The figure shows three views and two pictorial views of one solid part (mm, origin at its lowest corner). Answer the questions. A direction names the side the tool comes from. Coordinates: 2 decimals unless noted, no trailing zeros. Loops run counter-clockwise (first coordinate to the right, second up) from the corner with the lowest first, then second, coordinate; pieces in that order, holes last.
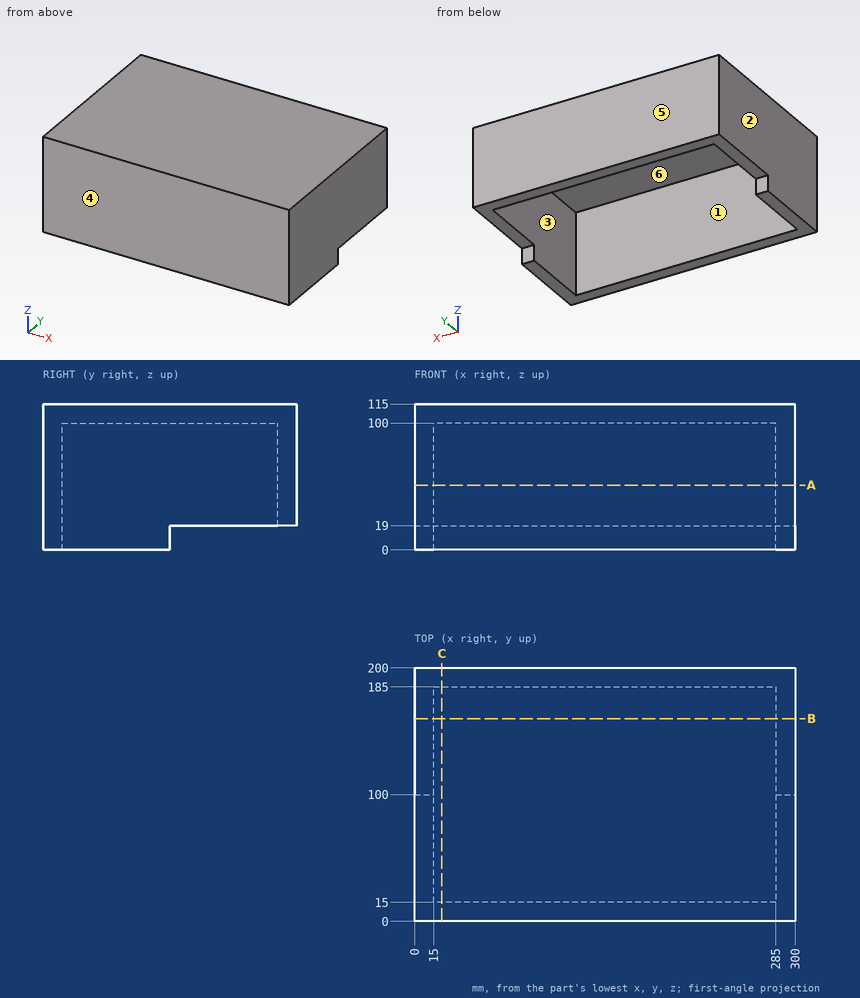
1. For the marked faces 5 and 6, determine the directions among +Z, -Z, +X, -X, +Y, -Y from which every point of the face is accessible in a straight line to the end or side of a thin tool.
2. Each of these flat-tipped pins is pushed along its axis until it touches: P1, Ø10, axis at x = 181, y = 79.5, coming from the -Z side; P2, Ø12, axis at x = 294, z = 5, coming from the +Y side. Where does it stop, or does it pass through?
3. A cutting plane is placed at B-B, the plane y = 160. Give the vertices of the cut face in (x, z), then the cut area to 3 significant figures.
4. A cutting plane is placed at A-A, the plane z = 51. Give the vertices of the cut face in (x, y), then the cut area to 3 significant figures.
5. Determine the mould class of the marked faces 1, 2, 3 and 4 for opening direction X: released by +X, released by -X, zero draft, split by the parting line, or undercut.
6. A cutting plane is placed at C-C, the plane x = 21.5. Give the vertices of the cut face in (y, z).
7. Straight lines are drawn through the part: probe 1 along Y at (x, z) = (19, 72.5); probe 2 along X at (y, z) = (100, 65.5); probe 3 along Z at (x, y) = (30, 73.5). For each, find the intervals that lie inside material, in ascending order.
Answers below:
1. face 5: +Z, -Z, +X, -X, +Y
1. face 6: -Z
2. P1: stops at z = 100
2. P2: stops at y = 100
3. outline: (0, 19) - (15, 19) - (15, 100) - (285, 100) - (285, 19) - (300, 19) - (300, 115) - (0, 115) - close
3. area: 6,930 mm2
4. outline: (0, 0) - (300, 0) - (300, 200) - (0, 200) - close; hole (15, 15) - (285, 15) - (285, 185) - (15, 185) - close
4. area: 14,100 mm2
5. face 1: undercut
5. face 2: released by -X
5. face 3: undercut
5. face 4: zero draft
6. outline: (0, 0) - (15, 0) - (15, 100) - (185, 100) - (185, 19) - (200, 19) - (200, 115) - (0, 115) - close
7. probe 1: y = 0 to 15, 185 to 200
7. probe 2: x = 0 to 15, 285 to 300
7. probe 3: z = 100 to 115
